For this review, use the dimensioned drawing (mm, ordinates from the lowest corner) and the shaded views. A direction names the side the tool comes from. Round coordinates to 2 decimals unless told otherwise and drop trailing zeros. Order: outer loops, then holes, each group sorted by start corner. A loop starts at its lowest first (then second) coordinate and runs counter-clockwise, first axis right, second up. Notation, with made-up numbers: M 28.5,43 L 78.5,43 A9 cw 78.5,50 Z; hole C 31.5,49 d9. An arc over 180 degrees is marked long. Use a Markdown table: item, result. Add a question column.
1. Consider section A-A on y = 12.75. State the section outline as (x, z) points, then the cut area to 3 significant figures.
2. Consider section C-C on z = 2.5. State the section outline as (x, y) points.
3. The part is to be moulded in two halves that separate along Y. For the marked faces 1, 2 and 3, say which applies: +Y half, -Y half, draft (parallel to the pull), parting line (faces both ways), or undercut.
4. Insertion check: P1, Ø1, axis at y = 19, z = 1, coming from the -X side. The pin has a flat end and moves straight along its axis. Give the tip position at first contact, or say it passes through.
5. Consider section D-D on x = 0.2. Count the separate pieces of the cut face and the enclosed holes in it, then the cut area to 3 significant figures.
6. Consider section B-B on z = 5. State the section outline as (x, y) points (1 decimal).
7. For the marked faces 4 and 5, list the 3-axis set-ups (+Z, -Z, +X, -X, +Y, -Y) from which the entire face can be reached by the end or side of a thin tool; tool diameter is ignored.
8. To check wall thickness, follow probe 1 along Y at (x, z) = (1.9, 3.5); probe 2 along Y at (x, z) = (0.8, 3) (1 decimal); probe 3 along Z at (x, y) = (1.3, 11.5). State the ranges of each line that lie inside material, in increasing order.
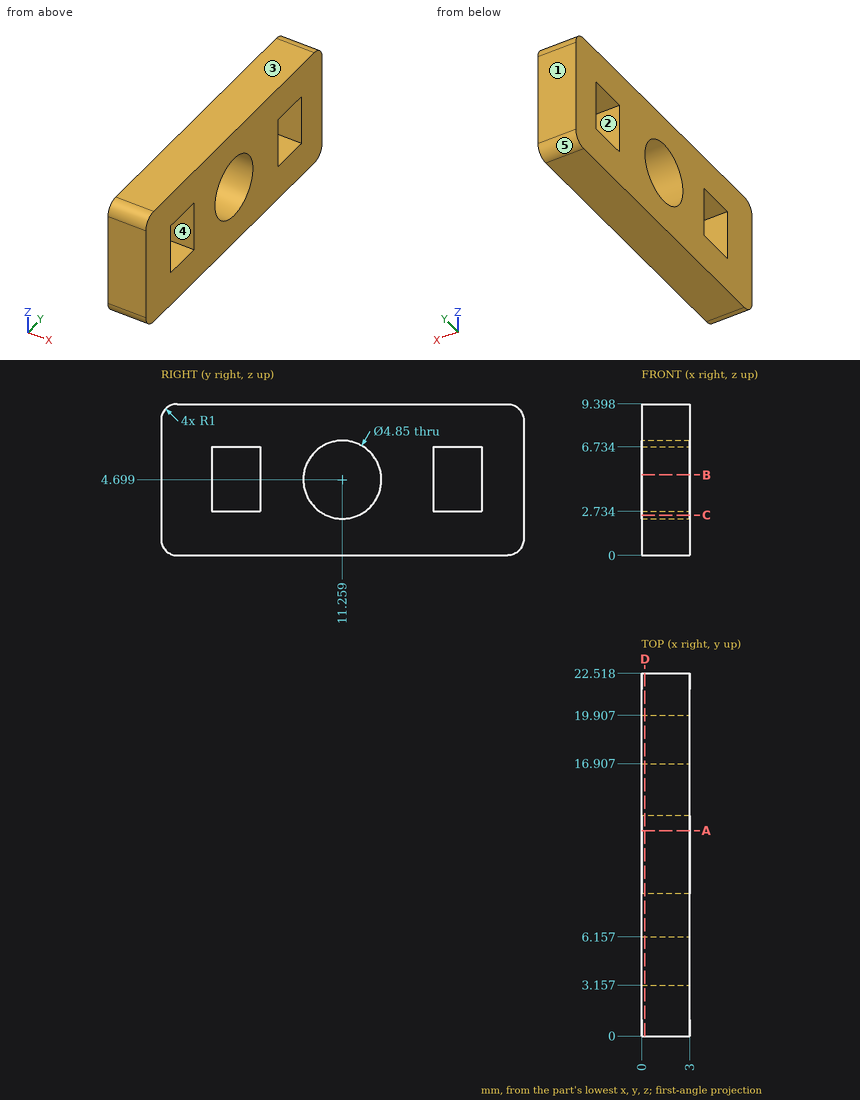
Answer block:
| question | item | result |
|---|---|---|
| 1 | outline | M 0,0 L 3,0 L 3,2.79 L 0,2.79 Z; M 0,6.61 L 3,6.61 L 3,9.4 L 0,9.4 Z |
| 1 | area | 16.7 mm^2 |
| 2 | outline | M 0,0 L 3,0 L 3,10.24 L 0,10.24 Z; M 0,12.28 L 3,12.28 L 3,22.52 L 0,22.52 Z |
| 3 | face 1 | +Y half |
| 3 | face 2 | undercut |
| 3 | face 3 | draft |
| 4 | P1 | x = 0 |
| 5 | separate pieces | 1 |
| 5 | enclosed holes | 3 |
| 5 | area | 168 mm^2 |
| 6 | outline | M 0,0 L 3,0 L 3,3.2 L 0,3.2 Z; M 0,6.2 L 3,6.2 L 3,8.9 L 0,8.9 Z; M 0,13.7 L 3,13.7 L 3,16.9 L 0,16.9 Z; M 0,19.9 L 3,19.9 L 3,22.5 L 0,22.5 Z |
| 7 | face 4 | +X, -X |
| 7 | face 5 | -Z, +X, -X, +Y |
| 8 | probe 1 | 0 to 3.16, 6.16 to 9.15, 13.37 to 16.91, 19.91 to 22.52 |
| 8 | probe 2 | 0 to 3.2, 6.2 to 9.5, 13 to 16.9, 19.9 to 22.5 |
| 8 | probe 3 | 0 to 2.29, 7.11 to 9.4 |
